```python
from build123d import *
from build123d.topology import SkipClean

# Parameters (mm, degrees)
EXTRUDE1_DEPTH      = 62.484
EXTRUDE1_DEPTH_BACK = 62.484
SKETCH1_R           = 19.05
SKETCH1_R_2         = 17.399
EXTRUDE2_DEPTH      = 62.484
EXTRUDE2_DEPTH_BACK = 62.484
SKETCH2_R           = 19.05
SKETCH2_R_2         = 17.399
EXTRUDE3_DEPTH      = 62.484
EXTRUDE3_DEPTH_BACK = 62.484
SKETCH3_R           = 19.05
SKETCH3_R_2         = 17.399
EXTRUDE4_START      = -81.534000101
EXTRUDE4_OUTLINE_R  = 17.399
EXTRUDE4_DEPTH      = 38.100000201
SKETCH5_R           = 17.399
EXTRUDE5_DEPTH      = 154.053917211
SKETCH6_R           = 17.399
EXTRUDE6_DEPTH      = 154.053917211
SKETCH7_R           = 34.925
SKETCH7_R_2         = 17.399
EXTRUDE7_DEPTH      = 12.7
SKETCH8_R           = 34.925
SKETCH8_R_2         = 17.399
EXTRUDE8_DEPTH      = 12.7
SKETCH9_R           = 34.925
SKETCH9_R_2         = 17.399
EXTRUDE9_DEPTH      = 12.7


# Read off the part's stored shape, not the designer's step: Extrude4
with BuildPart() as part:
    # Sketch1 → Extrude1 (new, two sides: drawn at the far end of the back side and taken through both)
    with BuildSketch(Plane(origin=(0, 0, 0), x_dir=(1, 0, 0), z_dir=(0, 1, 0)).offset(-EXTRUDE1_DEPTH_BACK)):
        with Locations(Location((0, 0, 0), (0, 0, 270))):
            Circle(SKETCH1_R)
        with Locations(Location((0, 0, 0), (0, 0, 270))):
            Circle(SKETCH1_R_2, mode=Mode.SUBTRACT)
    extrude(amount=EXTRUDE1_DEPTH + EXTRUDE1_DEPTH_BACK)

    # Sketch2 → Extrude2 (add, two sides: drawn at the far end of the back side and taken through both)
    with BuildSketch(Plane.XY.offset(-EXTRUDE2_DEPTH_BACK)):
        Circle(SKETCH2_R)
        Circle(SKETCH2_R_2, mode=Mode.SUBTRACT)
    extrude(amount=EXTRUDE2_DEPTH + EXTRUDE2_DEPTH_BACK)

    # Sketch3 → Extrude3 (add, two sides: drawn at the far end of the back side and taken through both)
    with BuildSketch(Plane(origin=(0, 0, 0), x_dir=(0, 0, -1), z_dir=(1, 0, 0)).offset(-EXTRUDE3_DEPTH_BACK)):
        Circle(SKETCH3_R)
        Circle(SKETCH3_R_2, mode=Mode.SUBTRACT)
    extrude(amount=EXTRUDE3_DEPTH + EXTRUDE3_DEPTH_BACK)

    # Extrude4 outline → Extrude4 (cut)
    with BuildSketch(Plane(origin=(62.484, 0, 0), x_dir=(0, 0, -1), z_dir=(1, 0, 0)).offset(EXTRUDE4_START)):
        Circle(EXTRUDE4_OUTLINE_R)
    extrude(amount=EXTRUDE4_DEPTH, mode=Mode.SUBTRACT)

    # Sketch5 → Extrude5 (cut, through all)
    with SkipClean():  # the faces are left unmerged after this step: merging them gives an invalid solid
        with BuildSketch(Plane(origin=(0, 0, -62.484), x_dir=(-1, 0, 0), z_dir=(0, 0, -1))):
            with Locations(Location((0, 0, 0), (0, 0, 180))):
                Circle(SKETCH5_R)
        extrude(amount=-EXTRUDE5_DEPTH, mode=Mode.SUBTRACT)

    # Sketch6 → Extrude6 (cut, through all)
    with BuildSketch(Plane(origin=(0, 62.484, 0), x_dir=(1, 0, 0), z_dir=(0, 1, 0))):
        with Locations(Location((0, 0, 0), (0, 0, 270))):
            Circle(SKETCH6_R)
    extrude(amount=-EXTRUDE6_DEPTH, mode=Mode.SUBTRACT)

    # Sketch7 → Extrude7 (add)
    with BuildSketch(Plane(origin=(62.484, 0, 0), x_dir=(0, 0, -1), z_dir=(1, 0, 0))):
        Circle(SKETCH7_R)
        Circle(SKETCH7_R_2, mode=Mode.SUBTRACT)
    extrude7 = extrude(amount=-EXTRUDE7_DEPTH)

    # Mirror1: Extrude7 across plane
    add(extrude7.mirror(Plane(origin=(0, 0, 0), x_dir=(0, 0, 1), z_dir=(1, 0, 0))))

    # Sketch8 → Extrude8 (add)
    with BuildSketch(Plane(origin=(0, 0, -62.484), x_dir=(-1, 0, 0), z_dir=(0, 0, -1))):
        Circle(SKETCH8_R)
        with Locations(Location((0, 0, 0), (0, 0, 180))):
            Circle(SKETCH8_R_2, mode=Mode.SUBTRACT)
    extrude8 = extrude(amount=-EXTRUDE8_DEPTH)

    # Mirror2: Extrude8 across plane
    add(extrude8.mirror(Plane.XY))

    # Sketch9 → Extrude9 (add)
    with BuildSketch(Plane(origin=(0, 62.484, 0), x_dir=(1, 0, 0), z_dir=(0, 1, 0))):
        with Locations(Location((0, 0, 0), (0, 0, 270))):
            Circle(SKETCH9_R)
        with Locations(Location((0, 0, 0), (0, 0, 270))):
            Circle(SKETCH9_R_2, mode=Mode.SUBTRACT)
    extrude9 = extrude(amount=-EXTRUDE9_DEPTH)

    # Mirror3: Extrude9 across plane
    add(extrude9.mirror(Plane.ZX))


solid = part.part
```
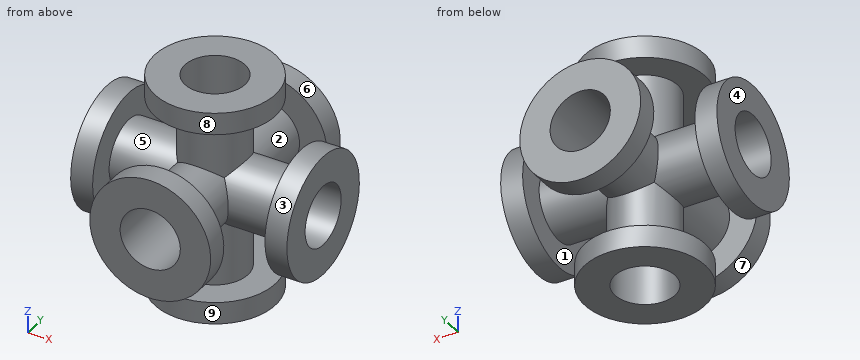
Design review of the part built by this model. Coordinates are the model's own, in mm. Face numbers are marked on the shaded views. A direction names the side the tool comes from. Coordinates: 2 decimals unless noted, no trailing zeros. Loops run counter-clockwise (first coordinate to the right, second up) from the corner with the lowest first, then second, coordinate; pieces in that order, holes last. Notation, with made-up numbers: (12, 85) -> (44, 85) arc R23 cw to (44, 118) -> close; hole circle Ø11 at (59, 70). An arc over 180 degrees is marked (long way). Answer as a JSON object with one key per item and string values.
Q1. To check wall thickness, follow L1, parallel to Y at x = 0, z = 46; L2, parallel to X at y = -27, z = 0; L3, parallel to Y at x = -2, z = -30.5. State the ranges of each line that lie inside material, in increasing order.
Answer block:
{"L1": "y = -19.05 to -17.4, 17.4 to 19.05", "L2": "x = -62.48 to -49.78, -19.05 to -17.4, 17.4 to 19.05, 49.78 to 62.48", "L3": "y = -62.48 to -49.78, -18.94 to -17.28, 17.28 to 18.94, 49.78 to 62.48"}
Q2. Take a section at A-A on x = -21. Give the boundary of the cut face in (y, z), plus the area to 3 significant figures.
Answer block:
{"outline": "(-62.48, -27.91) -> (-49.78, -27.91) -> (-49.78, 27.91) -> (-62.48, 27.91) -> close; (-27.91, -62.48) -> (27.91, -62.48) -> (27.91, -49.78) -> (-27.91, -49.78) -> close; (-27.91, 49.78) -> (27.91, 49.78) -> (27.91, 62.48) -> (-27.91, 62.48) -> close; circle Ø38.1 at (0, 0); (49.78, -27.91) -> (62.48, -27.91) -> (62.48, 27.91) -> (49.78, 27.91) -> close; hole circle Ø34.8 at (0, 0)", "area": "3,020 mm^2"}
Q3. Take a section at D-D on z = -48. Give the boundary of the cut face in (x, y).
Answer block:
{"outline": "circle Ø38.1 at (0, 0); hole circle Ø34.8 at (0, 0)"}
Q4. The part is to be moulded in two halves that separate along X. For the marked faces 1, 2, 3 and 4, say which applies: +X half, -X half, draft (parallel to the pull), parting line (faces both ways), or undercut.
Answer block:
{"face 1": "undercut", "face 2": "undercut", "face 3": "draft", "face 4": "-X half"}
Q5. Tool access review of the marked faces 5, 6, 7, 8 and 9: name each direction out of +Z, -Z, +X, -X, +Y, -Y from which nothing blocks a thin tool from reaching the whole face with its end or side.
Answer block:
{"face 5": "none", "face 6": "+Y", "face 7": "-Y", "face 8": "+Z", "face 9": "-Z"}
Q6. Take a section at B-B on y = 0. Give the number of separate pieces and of enclosed holes in the cut face, plus the area to 3 significant figures.
Answer block:
{"separate pieces": "4", "enclosed holes": "0", "area": "2,200 mm^2"}
Q7. Clearance check with flat-ended pins moving along their axes: pin 1 Ø3 at (x, z) = (45, 8) entering from +Y; pin 2 Ø2 at (x, y) = (45.5, -5.5) entering from -Z; pin 3 Ø12 at (x, z) = (-42.5, -44.5) entering from +Y; pin 4 Ø21 at (x, z) = (-7, 3) entering from -Y. State where each tip first meets the part, or that it passes through.
Answer block:
{"pin 1": "stops at y = 17.91", "pin 2": "stops at z = -18.51", "pin 3": "passes through", "pin 4": "stops at y = -62.48"}
